For this review, take the finished solid that the model builds, in its own axes (mm). Face numbers are marked on the shaded views. A direction names the side the tool comes from. Round coordinates to 2 decimals unless told otherwise and drop trailing zeros. Loops run counter-clockwise (first coordinate to the right, second up) from the corner with the lowest first, then second, coordinate; pieces in that order, holes last.
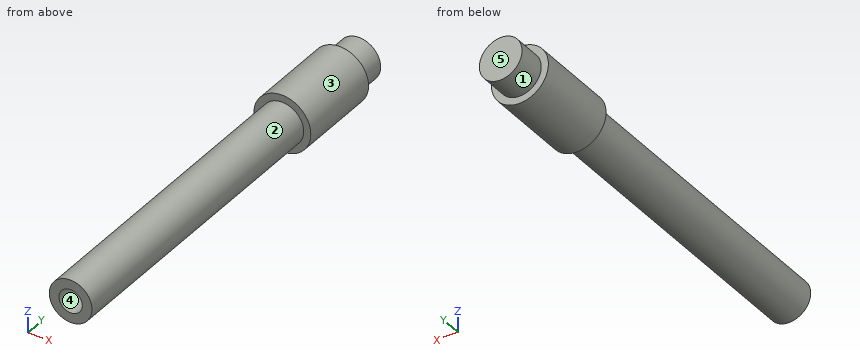
```python
from build123d import *

# Parameters (mm, degrees)
SKETCH2_R          = 4.1
CUT_EXTRUDE1_DEPTH = 50


with BuildPart() as part:
    # Sketch1 → Revolve1 (revolve)
    with BuildSketch(Plane.XY, mode=Mode.PRIVATE) as revolve1_sk:
        Polygon((0, -75), (0, 75), (-7.5, 75), (-7.5, 65), (-10, 65), (-10, 35), (-7.5, 35), (-7.5, -75), align=None)
    revolve(revolve1_sk.sketch.rotate(Axis((0, -75, 0), (0, 1, 0)), 180), axis=Axis((0, -75, 0), (0, 1, 0)))

    # Sketch2 → Cut-Extrude1 (cut)
    with BuildSketch(Plane.XZ.offset(75)):
        Circle(SKETCH2_R)
    extrude(amount=-CUT_EXTRUDE1_DEPTH, mode=Mode.SUBTRACT)


solid = part.part
```
(1) For the marked faces 1 and 2, list the 3-axis set-ups (+Z, -Z, +X, -X, +Y, -Y) from which the entire face can be reached by the end or side of a thin tool; tool diameter is ignored.
(2) Insertion check: pin 1 Ø5 at (y, z) = (-58.5, -0.5) entering from -X; pin 2 Ø12 at (y, z) = (-41, 2) entering from +X; pin 3 Ø4 at (x, y) = (5.5, -40) entering from +Z; pin 4 Ø9 at (x, z) = (2, 1) entering from -Y. Each pin has a flat end and moves straight along its axis. Give the tip position at first contact, or say it passes through.
(3) Add section D-D (y = -20). Give the boundary of the cut face in (x, z).
(4) Add section C-C (y = -63). Give the boundary of the cut face in (x, z), plus the area to 3 significant figures.
(5) The part is to be moulded in two halves that separate along Z. For the marked faces 3, 4 and 5, say which applies: pulls with the +Z half, pulls with the -Z half, needs draft (parallel to the pull), parting line crosses it, or undercut.
(6) Add section B-B (x = 0). Give the boundary of the cut face in (y, z), plus the area to 3 significant figures.
(7) Add section A-A (z = 0). Give the boundary of the cut face in (x, y).
(8) For L1, parallel to Z at x = 0, y = -37; L2, parallel to Y at x = -5.75, z = 5.25; L3, parallel to Y at x = 1.5, z = -2.75, list the stretches that pass through material, from the lowest coordinate up.
Outcome:
1. face 1: +Y
1. face 2: -Y
2. pin 1: stops at x = -7.5
2. pin 2: stops at x = 7.5
2. pin 3: stops at z = 6.63
2. pin 4: stops at y = -75
3. outline: circle Ø15 at (0, 0)
4. outline: circle Ø15 at (0, 0); hole circle Ø8.2 at (0, 0)
4. area: 124 mm2
5. face 3: parting line crosses it
5. face 4: undercut
5. face 5: needs draft
6. outline: (-75, -7.5) - (35, -7.5) - (35, -10) - (65, -10) - (65, -7.5) - (75, -7.5) - (75, 7.5) - (65, 7.5) - (65, 10) - (35, 10) - (35, 7.5) - (-75, 7.5) - (-75, 4.1) - (-25, 4.1) - (-25, -4.1) - (-75, -4.1) - close
6. area: 1,990 mm2
7. outline: (-10, 35) - (-7.5, 35) - (-7.5, -75) - (-4.1, -75) - (-4.1, -25) - (4.1, -25) - (4.1, -75) - (7.5, -75) - (7.5, 35) - (10, 35) - (10, 65) - (7.5, 65) - (7.5, 75) - (-7.5, 75) - (-7.5, 65) - (-10, 65) - close
8. L1: z = -7.5 to -4.1, 4.1 to 7.5
8. L2: y = 35 to 65
8. L3: y = -25 to 75
